Geometry check sheet. Reference: the model listing, model coordinates, mm. A direction names the side the tool comes from. Give positions to 0.01 mm unless a question says otherwise; leave off trailing zeros. Order: outer loops, then holes, each group sorted by start corner. A loop starts at its lowest first (then second) coordinate and runs counter-clockwise, first axis right, second up. Notation, with made-up numbers: M -24,-32.5 L -8,-32.5 A19 cw -8,-23.5 Z; hole C -14,8 d9. An arc over 180 degrees is marked long. Answer as CSV lines item,"result". Start each with the question number.
```python
from build123d import *

# Parameters (mm, degrees)
F1_DEPTH      = 88.9
F3_DEPTH      = 25.4
F3_DEPTH_BACK = 107.95
F4_R          = 11.176
F5_DEPTH      = 99.27772


with BuildPart() as f1:
    # F0 (on Front) → F1 (new body)
    with BuildSketch(Plane.XZ):
        with BuildLine():
            Line((93.508288, -49.63886), (93.508288, 49.63886))
            Line((93.508288, 49.63886), (58.457912, 49.63886))
            ThreePointArc((58.457912, 49.63886), (0, -8.819052), (-58.457912, 49.63886))
            Line((-58.457912, 49.63886), (-93.508288, 49.63886))
            Line((-93.508288, 49.63886), (-93.508288, -49.63886))
            Line((-93.508288, -49.63886), (93.508288, -49.63886))
        make_face()
    extrude(amount=F1_DEPTH)

    # F2 (on face) → F3 (join, two sides)
    with BuildSketch(Plane.XZ.offset(88.9)) as f3_sk:
        with BuildLine():
            Line((-38.644901, 49.63886), (-58.457912, 49.63886))
            ThreePointArc((-58.457912, 49.63886), (0, -8.819052), (58.457912, 49.63886))
            Line((58.457912, 49.63886), (38.644901, 49.63886))
            ThreePointArc((38.644901, 49.63886), (0, 10.993959), (-38.644901, 49.63886))
        make_face()
    extrude(amount=F3_DEPTH)
    extrude(f3_sk.sketch, amount=-F3_DEPTH_BACK)

    # F4 (on face) → F5 (cut, through all)
    with BuildSketch(Plane.XY.offset(49.63886)):
        with Locations((-75.9831, -44.45)):
            Circle(F4_R)
        with Locations((74.703217, -44.45)):
            Circle(F4_R)
    extrude(amount=-F5_DEPTH, mode=Mode.SUBTRACT)


solid = f1.part
```
Item 1: Depth check by flat-ended pin: pin 1 Ø1.5 at (x, z) = (75, 32) entering from -Y; pin 2 Ø18 at (x, y) = (-75.98, -44.45) entering from +Z; pin 3 Ø6 at (x, y) = (10, -24.5) entering from +Z. Enter the tip coordinate at first touch or a pass-through.
Item 2: Section check B-B on y = -44.45. Record the boundary of the cut face in (x, z), then the cut area to 3 significant figures.
Item 3: Section check D-D on z = -28.5. Record the boundary of the cut face in (x, y), then the cut area to 3 significant figures.
Item 4: Section check A-A on z = 32.5. Record the boundary of the cut face in (x, y), then the cut area to 3 significant figures.
Item 5: Scan lines: line 1 along X through (y, z) = (-45, -8); line 2 along Y through (x, z) = (43, -42); line 3 along X through (y, z) = (-41, 14.5). Record each from-to range of solid material in increasing order.
Item 6: Section check C-C on x = 0. Record the boundary of the cut face in (y, z), then the cut area to 3 significant figures.
Item 7: Draft check along Y on faces 1 (the face through (-1, -88.9, -10)), 2 (the face through (0.85, -48.558, 11.003)), 3 (the face through (-65.323, -41.093, 0.695)). Enter one of: pulls with the +Y half, pulls with the -Y half, needs draft (parallel to the pull), parting line crosses it, or undercut.
Item 8: Access from +Z, -Z, +X, -X, +Y, -Y to the whole of each face (thin tool, end or side, straight path). Record for faces 4 (the face through (-1.285, 9.392, -8.805)), 5 (the face through (93.508, -44, -1)), 6 (the face through (-1.285, -101.422, -8.805)).
Numbers:
1,pin 1,"y = -88.9"
1,pin 2,"through"
1,pin 3,"z = 13.25"
2,outline,"M -93.51,-49.64 L -87.16,-49.64 L -87.16,49.64 L -93.51,49.64 Z; M -64.81,-49.64 L 63.53,-49.64 L 63.53,49.64 L 38.64,49.64 A38.64 cw -38.64,49.64 L -64.81,49.64 Z; M 85.88,-49.64 L 93.51,-49.64 L 93.51,49.64 L 85.88,49.64 Z"
2,area,"11,800 mm2"
3,outline,"M -93.51,-88.9 L 93.51,-88.9 L 93.51,0 L -93.51,0 Z; hole C -75.98,-44.45 d22.35; hole C 74.7,-44.45 d22.35"
3,area,"15,800 mm2"
4,outline,"M -93.51,-88.9 L -55.89,-88.9 L -55.89,-114.3 L -34.64,-114.3 L -34.64,19.05 L -55.89,19.05 L -55.89,0 L -93.51,0 Z; M 34.64,-114.3 L 55.89,-114.3 L 55.89,-88.9 L 93.51,-88.9 L 93.51,0 L 55.89,0 L 55.89,19.05 L 34.64,19.05 Z; hole C -75.98,-44.45 d22.35; hole C 74.7,-44.45 d22.35"
4,area,"11,600 mm2"
5,line 1,"-93.51 to -87.15, -64.82 to 63.54, 85.87 to 93.51"
5,line 2,"-88.9 to 0"
5,line 3,"-93.51 to -86.61, -65.35 to -16.08, 16.08 to 64.07, 85.33 to 93.51"
6,outline,"M -114.3,-8.82 L -88.9,-8.82 L -88.9,-49.64 L 0,-49.64 L 0,-8.82 L 19.05,-8.82 L 19.05,10.99 L -114.3,10.99 Z"
6,area,"6,270 mm2"
7,face 1,"pulls with the -Y half"
7,face 2,"needs draft"
7,face 3,"undercut"
8,face 4,"-Z, +Y"
8,face 5,"+Z, -Z, +X, +Y, -Y"
8,face 6,"-Z, -Y"
